```python
from build123d import *

# Parameters (mm, degrees)
ESBO_O1_W                = 31
ESBO_O1_H                = 25.5
RESSALTO_EXTRUS_O1_DEPTH = 2
ESBO_O2_W                = 27.5
ESBO_O2_H                = 21.5
RESSALTO_EXTRUS_O2_DEPTH = 16.2
ESBO_O3_W                = 1
ESBO_O3_H                = 6.5
ESBO_O3_W_2              = 27.5
ESBO_O3_H_2              = 1
RESSALTO_EXTRUS_O3_DEPTH = 9.5
ESBO_O4_W                = 24
ESBO_O4_H                = 19
RESSALTO_EXTRUS_O4_DEPTH = 1
RESSALTO_EXTRUS_O5_DEPTH = 19


with BuildPart() as part:
    # Esboço1 → Ressalto-extrusão1 (new body)
    with BuildSketch(Plane.XY):
        Rectangle(ESBO_O1_W, ESBO_O1_H)
    extrude(amount=RESSALTO_EXTRUS_O1_DEPTH)

    # Esboço2 → Ressalto-extrusão2 (add)
    with BuildSketch(Plane.XY.offset(2)):
        Rectangle(ESBO_O2_W, ESBO_O2_H)
    extrude(amount=RESSALTO_EXTRUS_O2_DEPTH)

    # Esboço3 → Ressalto-extrusão3 (add)
    with BuildSketch(Plane.XY.offset(18.2)):
        with Locations((-12, 5.375)):
            Rectangle(ESBO_O3_W, ESBO_O3_H)
        with Locations((0, -5.375)):
            Rectangle(ESBO_O3_W, ESBO_O3_H)
        with Locations((0, 5.375)):
            Rectangle(ESBO_O3_W, ESBO_O3_H)
        with Locations((-12, -5.375)):
            Rectangle(ESBO_O3_W, ESBO_O3_H)
        Rectangle(ESBO_O3_W_2, ESBO_O3_H_2)
    extrude(amount=RESSALTO_EXTRUS_O3_DEPTH)

    # Esboço4 → Ressalto-extrusão4 (add)
    with BuildSketch(Plane(origin=(0, 0, 0), x_dir=(-1, 0, 0), z_dir=(0, 0, -1))):
        Rectangle(ESBO_O4_W, ESBO_O4_H)
    extrude(amount=RESSALTO_EXTRUS_O4_DEPTH)

    # Esboço5 → Ressalto-extrusão5 (add)
    with BuildSketch(Plane.XZ.offset(9.5)):
        with BuildLine():
            Line((8.024552065, -1), (-12, -1))
            ThreePointArc((-12, -1), (-10.442623617, -4.60271069), (-7.5, -7.2))
            ThreePointArc((-7.5, -7.2), (-0.218681889, -2.895700597), (8.024552065, -1))
        make_face()
    extrude(amount=-RESSALTO_EXTRUS_O5_DEPTH)


solid = part.part
```
CAD build for the part. Positions are in the model's coordinates, mm. A direction names the side the tool comes from. Coordinates: 2 decimals unless noted, no trailing zeros. Write each loop counter-clockwise with the first axis right and the second up, starting at its lowest first coordinate (ties: lowest second). Pieces come first, ordered by that corner, then holes.
(1) Two-plate mould, pull along Y, no slides. Class faces 1 (the face through (-12, -2.125, 23)), 2 (the face through (-12, 5, 27.7)), 3 (the face through (-3, 9.5, -2)): +Y half, -Y half, draft (parallel to the pull), parting line (faces both ways), or undercut.
(2) Cut at D-D, the plane z = 11.5. List the corners of the cut face in (x, y).
(3) Cut at C-C, the plane y = 4.25. List the corners of the cut face in (x, z), and give its area (3 significant figures).
(4) Cut at B-B, the plane z = 19. List the corners of the cut face in (x, y) (3 decimals), and give its area (3 significant figures).
(5) Drill centre lines: probe 1 along X at (y, z) = (1.5, 12.5); probe 2 along Y at (x, z) = (8, 14); probe 3 along Z at (x, y) = (10.5, 7.25). Where is each one in solid material? Low to high.
(6) Flat gauge pins, fed straight in: pin 1 (8 mm diameter, centred on x = 3.5, y = -5.5, fed in from +Z); pin 2 (11 mm diameter, centred on y = -4, z = 19.5, fed in from -X); pin 3 (3 mm diameter, centred on x = 11.5, z = 22, fed in from -Y); pin 4 (4 mm diameter, centred on x = -8.5, y = 6, fed in from -Z). Where does each tip first touch, or does it go through?
(7) Cut at A-A, the plane x = 10.5. List the corners of the cut face in (y, z), and give its area (3 significant figures).
(8) 3-axis set-ups, long thin cutter, end or side, ignore diameter. For faces 4 (the face through (-0.5, -5, 23)), 5 (the face through (0.5, 5, 23)), 6 (the face through (-12.5, -5, 23)), 7 (the face through (10, 0, -1)), 8 (the face through (0, -2.125, 23)): which of +Z, -Z, +X, -X, +Y, -Y reach the whole face in a straight line?
Geometry says:
1. face 1: undercut
1. face 2: draft
1. face 3: +Y half
2. outline: (-13.75, -10.75) - (13.75, -10.75) - (13.75, 10.75) - (-13.75, 10.75) - close
3. outline: (-15.5, 0) - (-12, 0) - (-12, -1) arc R9 ccw to (-7.5, -7.2) arc R27.59 cw to (8.02, -1) - (12, -1) - (12, 0) - (15.5, 0) - (15.5, 2) - (13.75, 2) - (13.75, 18.2) - (0.5, 18.2) - (0.5, 27.7) - (-0.5, 27.7) - (-0.5, 18.2) - (-11.5, 18.2) - (-11.5, 27.7) - (-12.5, 27.7) - (-12.5, 18.2) - (-13.75, 18.2) - (-13.75, 2) - (-15.5, 2) - close
3. area: 602 mm2
4. outline: (-13.75, -0.5) - (13.75, -0.5) - (13.75, 0.5) - (-13.75, 0.5) - close; (-12.5, -8.625) - (-11.5, -8.625) - (-11.5, -2.125) - (-12.5, -2.125) - close; (-12.5, 2.125) - (-11.5, 2.125) - (-11.5, 8.625) - (-12.5, 8.625) - close; (-0.5, -8.625) - (0.5, -8.625) - (0.5, -2.125) - (-0.5, -2.125) - close; (-0.5, 2.125) - (0.5, 2.125) - (0.5, 8.625) - (-0.5, 8.625) - close
4. area: 53.5 mm2
5. probe 1: x = -13.75 to 13.75
5. probe 2: y = -10.75 to 10.75
5. probe 3: z = -1 to 18.2
6. pin 1: stops at z = 27.7
6. pin 2: stops at x = -13.75
6. pin 3: stops at y = -0.5
6. pin 4: stops at z = -7.2
7. outline: (-12.75, 0) - (-9.5, 0) - (-9.5, -1) - (9.5, -1) - (9.5, 0) - (12.75, 0) - (12.75, 2) - (10.75, 2) - (10.75, 18.2) - (0.5, 18.2) - (0.5, 27.7) - (-0.5, 27.7) - (-0.5, 18.2) - (-10.75, 18.2) - (-10.75, 2) - (-12.75, 2) - close
7. area: 428 mm2
8. face 4: +Z, -Y
8. face 5: +Z, +X, +Y
8. face 6: +Z, -X, -Y
8. face 7: -Z, +X, +Y, -Y
8. face 8: +Z, +X, -X
